Autodesk Inventor part; units mm, degrees
ref_plane "YZ Plane" through (0, 0, 0) normal (1, 0, 0) x (0, 1, 0)
ref_plane "XZ Plane" through (0, 0, 0) normal (0, 1, 0) x (-1, 0, 0)
ref_plane "XY Plane" through (0, 0, 0) normal (0, 0, 1) x (1, 0, 0)
sketch "Sketch1" plane through (0, 0, 0) normal (0, 0, 1) x (1, 0, 0)
  line L0 (1.4665, -2.54) -> (-1.4665, -2.54)
  line L1 (-1.4665, -2.54) -> (-2.9329, 0)
  line L2 (-2.9329, 0) -> (-1.4665, 2.54)
  line L3 (-1.4665, 2.54) -> (1.4665, 2.54)
  line L4 (1.4665, 2.54) -> (2.9329, 0)
  line L5 (2.9329, 0) -> (1.4665, -2.54)
  point P0 (0, 0)
  point P1 (0, 0)
  point P2 (0, -2.54)
  dimension "d1" = 2.54
  dimension "d2" = 2.54
extrude "Extrusion1" add sketch "Sketch1" along normal blind 2
sketch "Sketch2" plane through (0, 0, 2) normal (0, 0, 1) x (1, 0, 0)
  circle A0 centre (0, 0) radius 1.5
  dimension "d5" = 3
extrude "Extrusion2" add sketch "Sketch2" along normal blind 6
thread "Thread1"
properties part number "M3 screw_6mm"
CAD build for the part. Positions are in the model's coordinates, mm. A direction names the side the tool comes from. Round coordinates to 2 decimals unless told otherwise and drop trailing zeros. Write each loop counter-clockwise with the first axis right and the second up, starting at its lowest first coordinate (ties: lowest second). Pieces come first, ordered by that corner, then holes.
(1) 3-axis set-ups, long thin cutter, end or side, ignore diameter. For faces 1 (the face through (1.3, 1.2, 2)), 2 (the face through (0, 2.54, 1)): which of +Z, -Z, +X, -X, +Y, -Y reach the whole face in a straight line?
(2) Probe line 1 along Z through (x, y) = (1.65, 0.8); line 2 along X through (y, z) = (0.05, 3.5); line 3 along X through (y, z) = (0.65, 3.5). List the from-to ranges inside material, lowest first.
(3) Drop flat-ended pins along their axis: P1, Ø1.5, axis at x = -2.5, y = 1.5, coming from the +Z side; P2, Ø3, axis at x = -1, z = 4, coming from the +Y side; P3, Ø1.5, axis at x = 1.5, z = 5, coming from the +Y side. Give the stop position or say it passes through.
(4) Slice it at D-D, the plane z = 4.25. Write the cut outline in (x, y).
(5) Slice it at C-C, the plane y = 0.9. Write the cut outline in (x, z), and give its area (3 significant figures).
(6) Slice it at A-A, the plane x = 0. Write the cut outline in (y, z).
(7) Slice it at B-B, the plane z = 1.5. Write the cut outline in (x, y).
From the geometry:
1. face 1: +Z
1. face 2: +Z, -Z, +X, -X, +Y
2. line 1: z = 0 to 2
2. line 2: x = -1.5 to 1.5
2. line 3: x = -1.35 to 1.35
3. P1: stops at z = 2
3. P2: stops at y = 1.5
3. P3: stops at y = 1.3
4. outline: circle Ø3 at (0, 0)
5. outline: (-2.41, 0) - (2.41, 0) - (2.41, 2) - (1.2, 2) - (1.2, 8) - (-1.2, 8) - (-1.2, 2) - (-2.41, 2) - close
5. area: 24.1 mm2
6. outline: (-2.54, 0) - (2.54, 0) - (2.54, 2) - (1.5, 2) - (1.5, 8) - (-1.5, 8) - (-1.5, 2) - (-2.54, 2) - close
7. outline: (-2.93, 0) - (-1.47, -2.54) - (1.47, -2.54) - (2.93, 0) - (1.47, 2.54) - (-1.47, 2.54) - close
